Build history of the part. All positions in model axes, mm. A direction names the side the tool comes from. Coordinates: 2 decimals unless noted, no trailing zeros. One line per item, written item: value.
```python
from build123d import *

# Parameters (mm, degrees)
SKETCH1_W           = 68
SKETCH1_H           = 46
BOSS_EXTRUDE1_DEPTH = 3
SKETCH2_W           = 64
SKETCH2_H           = 42
CUT_EXTRUDE1_DEPTH  = 2
SNAP_START          = 17.5
SNAP_HOOK1_DEPTH    = 3
SNAP_START_2        = -10.5
SNAP_HOOK2_DEPTH    = 3
FILLET3_R           = 3
FILLET4_R           = 3
FILLET5_R           = 3
SKETCH4_W           = 2.752193097
SKETCH4_H           = 4.417994182
CUT_EXTRUDE2_DEPTH  = 1


# Read off the part's stored shape, not the designer's step: Snap Hook1, Snap Hook2
# Some blends are built 0.0001 mm under size
with BuildPart() as part:
    # Sketch1 → Boss-Extrude1 (new body)
    with BuildSketch(Plane(origin=(0, 0, 0), x_dir=(1, 0, 0), z_dir=(0, 1, 0))):
        Rectangle(SKETCH1_W, SKETCH1_H)
    extrude(amount=BOSS_EXTRUDE1_DEPTH)

    # Sketch2 → Cut-Extrude1 (cut)
    with BuildSketch(Plane(origin=(0, 3, 0), x_dir=(1, 0, 0), z_dir=(0, 1, 0))):
        Rectangle(SKETCH2_W, SKETCH2_H)
    extrude(amount=-CUT_EXTRUDE1_DEPTH, mode=Mode.SUBTRACT)

    # Snap Hook1 outline → Snap Hook1 (add)
    with BuildSketch(Plane.YZ.offset(SNAP_START)):
        Polygon((5, -21.5), (5.2, -21), (5.2, -20.2), (1, -19), (1, -21), (4.5, -21), (4.5, -21.5), align=None)
    snap_hook1 = extrude(amount=SNAP_HOOK1_DEPTH)

    # Snap Hook2 outline → Snap Hook2 (add)
    with BuildSketch(Plane.YZ.offset(SNAP_START_2)):
        Polygon((5, -21.5), (5.2, -21), (5.2, -20.2), (1, -19), (1, -21), (4.5, -21), (4.5, -21.5), align=None)
    snap_hook2 = extrude(amount=SNAP_HOOK2_DEPTH)

    # Mirror1: Snap Hook1, Snap Hook2 across plane
    add(snap_hook1.mirror(Plane.XY))
    add(snap_hook2.mirror(Plane.XY))

    # Fillet3
    fillet3_edges = [part.edges().sort_by_distance(p)[0] for p in [
        (0, 0, -23),
        (34, 0, 0),
        (0, 0, 23),
        (-34, 0, 0),
    ]]
    fillet(fillet3_edges, radius=FILLET3_R - 0.0001)  # a hair under: the kernel refuses the full size

    # Fillet4
    # the kernel refuses this fillet: 3 mm, written as the material it takes off along each edge
    with BuildSketch(Plane(origin=(31, 0, 20), x_dir=(1, 0, 0), z_dir=(0, 0, -1))) as fillet4_piece_1:
        with BuildLine():
            CenterArc((0.0001, -2.9999), 2.9999, 0, 90)
            Line((3, -2.9999), (3, 0))
            Line((3, 0), (0.0001, 0))
        make_face()
    revolve(axis=Axis((31, 0, 20), (0, -1, 0)), revolution_arc=90, mode=Mode.SUBTRACT)
    with BuildSketch(Plane(origin=(-31, 0, 20), x_dir=(0, 0, 1), z_dir=(1, 0, 0))) as fillet4_piece_2:
        with BuildLine():
            CenterArc((0.0001, -2.9999), 2.9999, 0, 90)
            Line((3, -2.9999), (3, 0))
            Line((3, 0), (0.0001, 0))
        make_face()
    revolve(axis=Axis((-31, 0, 20), (0, -1, 0)), revolution_arc=90, mode=Mode.SUBTRACT)
    with BuildSketch(Plane(origin=(31, 0, -20), x_dir=(0, 0, -1), z_dir=(-1, 0, 0))) as fillet4_piece_3:
        with BuildLine():
            CenterArc((0.0001, -2.9999), 2.9999, 0, 90)
            Line((3, -2.9999), (3, 0))
            Line((3, 0), (0.0001, 0))
        make_face()
    revolve(axis=Axis((31, 0, -20), (0, -1, 0)), revolution_arc=90, mode=Mode.SUBTRACT)
    with BuildSketch(Plane(origin=(-31, 0, -20), x_dir=(-1, 0, 0), z_dir=(0, 0, 1))) as fillet4_piece_4:
        with BuildLine():
            CenterArc((0.0001, -2.9999), 2.9999, 0, 90)
            Line((3, -2.9999), (3, 0))
            Line((3, 0), (0.0001, 0))
        make_face()
    revolve(axis=Axis((-31, 0, -20), (0, -1, 0)), revolution_arc=90, mode=Mode.SUBTRACT)
    with BuildSketch(Plane(origin=(-34, 0, -23), x_dir=(0, 0, 1), z_dir=(0, 1, 0)), Plane(origin=(-34, 0, 23), x_dir=(1, 0, 0), z_dir=(0, 1, 0))) as fillet4_piece_5:
        with BuildLine():
            CenterArc((FILLET4_R, FILLET4_R), FILLET4_R, 180, 90)
            Line((0, FILLET4_R), (0, 0))
            Line((0, 0), (FILLET4_R, 0))
        make_face()
    extrude(amount=10.5, mode=Mode.SUBTRACT)
    with BuildSketch(Plane(origin=(34, 0, -23), x_dir=(0, 0, 1), z_dir=(0, 1, 0)), Plane(origin=(34, 0, 23), x_dir=(-1, 0, 0), z_dir=(0, 1, 0))) as fillet4_piece_6:
        with BuildLine():
            CenterArc((FILLET4_R, -FILLET4_R), FILLET4_R, 90, 90)
            Line((0, -FILLET4_R), (0, 0))
            Line((0, 0), (FILLET4_R, 0))
        make_face()
    extrude(amount=10.5, mode=Mode.SUBTRACT)

    # Fillet5
    fillet5_edges = [part.edges().sort_by_distance(p)[0] for p in [
        (-32, 2, 21),
        (-32, 2, -21),
        (32, 2, -21),
        (32, 2, 21),
    ]]
    fillet(fillet5_edges, radius=FILLET5_R)

    # Sketch4 → Cut-Extrude2 (cut)
    with BuildSketch(Plane(origin=(0, 3, 0), x_dir=(1, 0, 0), z_dir=(0, 1, 0))):
        with Locations((33.0987433, 0)):
            Rectangle(SKETCH4_W, SKETCH4_H)
    extrude(amount=-CUT_EXTRUDE2_DEPTH, mode=Mode.SUBTRACT)


solid = part.part
```
Item 1: Tool access for faces 1 (the face through (-33.14, 0.9, -0.28)), 2 (the face through (-10.5, 3, 20)), 3 (the face through (19, 4, -21)): list every direction of +Z, -Z, +X, -X, +Y, -Y with a clear straight run to the whole face (end or side of a thin tool).
Check result:
face 1: +Z, -Z, -X, -Y
face 2: +Y
face 3: -Z, +X, -X
Item 2: Probe probe 1 along X at (y, z) = (2.95, -9); probe 2 along Z at (x, y) = (28, 2.7); probe 3 along Y at (x, z) = (-31, 14.5). List the from-to ranges inside material, lowest first. Write a range as from..to.
Check result:
probe 1: x = -34..-32, 32..34
probe 2: z = -22.98..-21, 21..22.98
probe 3: y = 0..1
Item 3: Pull direction Z, two halves, no side cores. Call faces 4 (the face through (31.14, 1.99, -20.1)), 5 (the face through (-9, 4, 21)), 6 (the face through (0.43, 0.9, -22.14)), 7 (the face through (33.14, 0.9, -0.28)): released by +Z, released by -Z, zero draft, split by the parting line, or undercut.
Check result:
face 4: undercut
face 5: released by +Z
face 6: released by -Z
face 7: zero draft
Item 4: Drop flat-ended pins along their axis: P1, Ø0.8, axis at x = 18.5, y = 3.5, coming from the +Z side; P2, Ø8, axis at x = -24.5, z = 9, coming from the +Y side; P3, Ø1.6, axis at x = -17, y = 1.5, coming from the +Z side. Give the stop position or say it passes through.
Check result:
P1: stops at z = 21
P2: stops at y = 1
P3: stops at z = 22.92
